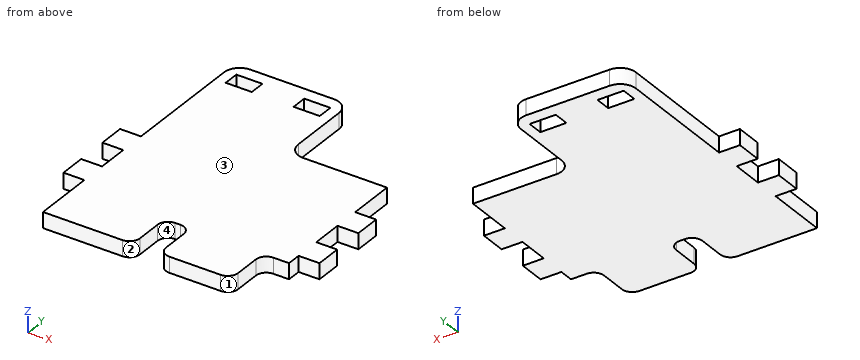
```python
from build123d import *

# Parameters (mm, degrees)
SKETCH_1_W          = 41
SKETCH_1_H          = 30
EXTRUDE_1_DEPTH     = 3
SKETCH_2_W          = 4
SKETCH_2_H          = 5
EXTRUDE_2_DEPTH     = 3
SKETCH_3_W          = 22
SKETCH_3_H          = 17.5
EXTRUDE_3_DEPTH     = 3
SKETCH_4_W          = 5
SKETCH_4_H          = 3
CUT_EXTRUDE_1_DEPTH = 10
SKETCH_5_W          = 41
SKETCH_5_H          = 6.7
EXTRUDE_4_DEPTH     = 3
SKETCH_6_W          = 5
SKETCH_6_H          = 9
CUT_EXTRUDE_2_DEPTH = 10
FILLET_1_R          = 3
FILLET_2_R          = 2


with BuildPart() as part:
    # 草图1 → 凸台-拉伸1 (new body)
    with BuildSketch(Plane.XY):
        Rectangle(SKETCH_1_W, SKETCH_1_H)
    extrude(amount=EXTRUDE_1_DEPTH)

    # 草图2 → 凸台-拉伸2 (add)
    with BuildSketch(Plane.XY.offset(3)):
        with Locations((22.5, -7.5)):
            Rectangle(SKETCH_2_W, SKETCH_2_H)
        with Locations((22.5, 3.5)):
            Rectangle(SKETCH_2_W, SKETCH_2_H)
        with Locations((-22.5, -7.5)):
            Rectangle(SKETCH_2_W, SKETCH_2_H)
        with Locations((-22.5, 3.5)):
            Rectangle(SKETCH_2_W, SKETCH_2_H)
    extrude(amount=-EXTRUDE_2_DEPTH)

    # 草图3 → 凸台-拉伸3 (add)
    with BuildSketch(Plane(origin=(0, 0, 0), x_dir=(-1, 0, 0), z_dir=(0, 0, -1))):
        with Locations((9.5, 23.75)):
            Rectangle(SKETCH_3_W, SKETCH_3_H)
    extrude(amount=-EXTRUDE_3_DEPTH)

    # 草图4 → 切除-拉伸1 (cut)
    with BuildSketch(Plane(origin=(0, 0, 0), x_dir=(-1, 0, 0), z_dir=(0, 0, -1))):
        with Locations((3, 28.5)):
            Rectangle(SKETCH_4_W, SKETCH_4_H)
        with Locations((16, 28.5)):
            Rectangle(SKETCH_4_W, SKETCH_4_H)
    extrude(amount=-CUT_EXTRUDE_1_DEPTH, mode=Mode.SUBTRACT)

    # 草图5 → 凸台-拉伸4 (add)
    with BuildSketch(Plane(origin=(0, 0, 0), x_dir=(-1, 0, 0), z_dir=(0, 0, -1))):
        with Locations((0, -18.35)):
            Rectangle(SKETCH_5_W, SKETCH_5_H)
    extrude(amount=-EXTRUDE_4_DEPTH)

    # 草图6 → 切除-拉伸2 (cut)
    with BuildSketch(Plane(origin=(0, 0, 0), x_dir=(-1, 0, 0), z_dir=(0, 0, -1))):
        with Locations((0.8, -17.2)):
            Rectangle(SKETCH_6_W, SKETCH_6_H)
        with Locations((-18, -17.2)):
            Rectangle(SKETCH_6_W, SKETCH_6_H)
    extrude(amount=-CUT_EXTRUDE_2_DEPTH, mode=Mode.SUBTRACT)

    # 圆角1
    fillet_1_edges = [part.edges().sort_by_distance(p)[0] for p in [
        (-20.5, 32.5, 1.5),
        (1.5, 15, 1.5),
        (1.5, 32.5, 1.5),
    ]]
    fillet(fillet_1_edges, radius=FILLET_1_R)

    # 圆角2
    fillet_2_edges = [part.edges().sort_by_distance(p)[0] for p in [
        (1.7, -21.7, 1.5),
        (-3.3, -21.7, 1.5),
        (15.5, -21.7, 1.5),
        (15.5, -12.7, 1.5),
        (1.7, -12.7, 1.5),
        (-3.3, -12.7, 1.5),
    ]]
    fillet(fillet_2_edges, radius=FILLET_2_R)


solid = part.part
```
The model under review builds one solid part; all positions refer to its coordinate system, in mm. Face numbers are marked on the shaded views. Round coordinates to 2 decimals unless told otherwise and drop trailing zeros. Order: outer loops, then holes, each group sorted by start corner. A loop starts at its lowest first (then second) coordinate and runs counter-clockwise, first axis right, second up.
Item 1: Add section A-A, the plane x = -15.5. State the section outline as (y, z) points.
Working result:
outline: (-21.7, 0) - (27, 0) - (27, 3) - (-21.7, 3) - close; (30, 0) - (32.5, 0) - (32.5, 3) - (30, 3) - close
Item 2: Add section C-C, the plane y = 28.5. State the section outline as (x, z) points.
Working result:
outline: (-20.5, 0) - (-18.5, 0) - (-18.5, 3) - (-20.5, 3) - close; (-13.5, 0) - (-5.5, 0) - (-5.5, 3) - (-13.5, 3) - close; (-0.5, 0) - (1.5, 0) - (1.5, 3) - (-0.5, 3) - close
Item 3: For pin 1 (1.5 mm diameter, centred on x = 9, z = 1, fed in from +Y); pin 2 (1 mm diameter, centred on x = 8.5, y = 15, fed in from -Z); pin 3 (1.5 mm diameter, centred on x = 19.5, z = 2, fed in from -Y); pin 4 (1.5 mm diameter, centred on x = 22, z = 1, fed in from -Y), all flat-tipped, find the tip position at first contact; note any pin that passes through.
Working result:
pin 1: stops at y = 15
pin 2: stops at z = 0
pin 3: stops at y = -12.7
pin 4: stops at y = -10
Item 4: Draft analysis for pull direction X (two halves, no side actions). For the marked faces 1, 2, 3 and 4, state which applies: released by +X, released by -X, zero draft, split by the parting line, or undercut.
Working result:
face 1: released by +X
face 2: undercut
face 3: zero draft
face 4: undercut
Item 5: Add section B-B, the plane y = -17. State the section outline as (x, z) points, and give its area (3 significant figures).
Working result:
outline: (-20.5, 0) - (-3.3, 0) - (-3.3, 3) - (-20.5, 3) - close; (1.7, 0) - (15.5, 0) - (15.5, 3) - (1.7, 3) - close
area: 93.0 mm2
Item 6: Add section D-D, the plane z = 2.1. Count the separate pieces of the cut face and the enclosed holes in it, and give its area (3 significant figures).
Working result:
separate pieces: 1
enclosed holes: 2
area: 1,850 mm2
Item 7: To check wall thickness, follow probe 1 along X at (y, z) = (28.5, 2); probe 2 along X at (y, z) = (-17, 1.15); probe 3 along X at (y, z) = (26, 1.5). State the ranges of each line that lie inside material, in increasing order.
Working result:
probe 1: x = -20.5 to -18.5, -13.5 to -5.5, -0.5 to 1.5
probe 2: x = -20.5 to -3.3, 1.7 to 15.5
probe 3: x = -20.5 to 1.5
